```python
from build123d import *

# Parameters (mm, degrees)
SKETCH1_W           = 7.3
SKETCH1_H           = 7.3
BOSS_EXTRUDE1_DEPTH = 1
BOSS_EXTRUDE2_DEPTH = 3
BOSS_EXTRUDE3_DEPTH = 1


with BuildPart() as part:
    # Sketch1 → Boss-Extrude1 (new body)
    with BuildSketch(Plane(origin=(0, 0, 0), x_dir=(1, 0, 0), z_dir=(0, 1, 0))):
        with BuildLine():
            Line((-6, -9), (6, -9))
            ThreePointArc((6, -9), (8.121320344, -8.121320344), (9, -6))
            Line((9, -6), (9, 6))
            ThreePointArc((9, 6), (8.121320344, 8.121320344), (6, 9))
            Line((6, 9), (-6, 9))
            ThreePointArc((-6, 9), (-8.121320344, 8.121320344), (-9, 6))
            Line((-9, 6), (-9, -6))
            ThreePointArc((-9, -6), (-8.121320344, -8.121320344), (-6, -9))
        make_face()
        Rectangle(SKETCH1_W, SKETCH1_H, mode=Mode.SUBTRACT)
    extrude(amount=BOSS_EXTRUDE1_DEPTH)

    # Sketch2 → Boss-Extrude2 (add)
    with BuildSketch(Plane(origin=(0, 1, 0), x_dir=(1, 0, 0), z_dir=(0, 1, 0))):
        with BuildLine():
            Line((-6, -9), (6, -9))
            ThreePointArc((6, -9), (8.121320344, -8.121320344), (9, -6))
            Line((9, -6), (9, 6))
            ThreePointArc((9, 6), (8.121320344, 8.121320344), (6, 9))
            Line((6, 9), (-6, 9))
            ThreePointArc((-6, 9), (-8.121320344, 8.121320344), (-9, 6))
            Line((-9, 6), (-9, -6))
            ThreePointArc((-9, -6), (-8.121320344, -8.121320344), (-6, -9))
        make_face()
        Polygon((-3.05, -3.65), (-3.05, -7.8), (3.05, -7.8), (3.05, -3.65), (3.65, -3.65), (3.65, -3.05), (7.8, -3.05), (7.8, 3.05), (3.65, 3.05), (3.65, 3.65), (3.05, 3.65), (3.05, 7.8), (-3.05, 7.8), (-3.05, 3.65), (-3.65, 3.65), (-3.65, 3.05), (-7.8, 3.05), (-7.8, -3.05), (-3.65, -3.05), (-3.65, -3.65), align=None, mode=Mode.SUBTRACT)
    extrude(amount=BOSS_EXTRUDE2_DEPTH)

    # Sketch3 → Boss-Extrude3 (add)
    with BuildSketch(Plane(origin=(0, 4, 0), x_dir=(1, 0, 0), z_dir=(0, 1, 0))):
        with BuildLine():
            Line((-3.65, -3.05), (-3.65, -3.65))
            Line((-3.65, -3.65), (-3.05, -3.65))
            Line((-3.05, -3.65), (-3.05, -9))
            Line((-3.05, -9), (-6, -9))
            ThreePointArc((-6, -9), (-8.121320344, -8.121320344), (-9, -6))
            Line((-9, -6), (-9, -3.05))
            Line((-9, -3.05), (-3.65, -3.05))
        make_face()
        with BuildLine():
            Line((6, -9), (3.05, -9))
            Line((3.05, -9), (3.05, -3.65))
            Line((3.05, -3.65), (3.65, -3.65))
            Line((3.65, -3.65), (3.65, -3.05))
            Line((3.65, -3.05), (9, -3.05))
            Line((9, -3.05), (9, -6))
            ThreePointArc((9, -6), (8.121320344, -8.121320344), (6, -9))
        make_face()
        with BuildLine():
            Line((3.65, 3.05), (3.65, 3.65))
            Line((3.65, 3.65), (3.05, 3.65))
            Line((3.05, 3.65), (3.05, 9))
            Line((3.05, 9), (6, 9))
            ThreePointArc((6, 9), (8.121320344, 8.121320344), (9, 6))
            Line((9, 6), (9, 3.05))
            Line((9, 3.05), (3.65, 3.05))
        make_face()
        with BuildLine():
            Line((-6, 9), (-3.05, 9))
            Line((-3.05, 9), (-3.05, 3.65))
            Line((-3.05, 3.65), (-3.65, 3.65))
            Line((-3.65, 3.65), (-3.65, 3.05))
            Line((-3.65, 3.05), (-9, 3.05))
            Line((-9, 3.05), (-9, 6))
            ThreePointArc((-9, 6), (-8.121320344, 8.121320344), (-6, 9))
        make_face()
    extrude(amount=BOSS_EXTRUDE3_DEPTH)


solid = part.part
```
The listing builds one solid part. Answer for the finished solid, in the listing's coordinates (mm). A direction names the side the tool comes from. Coordinates: 2 decimals unless noted, no trailing zeros. Loops run counter-clockwise (first coordinate to the right, second up) from the corner with the lowest first, then second, coordinate; pieces in that order, holes last. Notation, with made-up numbers: (3.25, 74.5) -> (33.25, 74.5) arc R18 ccw to (33.25, 80.5) -> close; hole circle Ø8 at (46.5, -21.5). An arc over 180 degrees is marked (long way). Use one line per item in the form item = value. Start each with the question number.
Item 1: The part is cut by section A-A on z = 0.5. Determine the outline of the cut face in (x, y), then the cut area to 3 significant figures.
Item 2: The part is cut by section D-D on y = 0.5. Determine the outline of the cut face in (x, z), then the cut area to 3 significant figures.
Item 3: The mould has two halves that part along X. Classify faces 5 (the face through (0, 2, 9)), 6 (the face through (0, 1, -6)), 7 (the face through (0, 4, 8)), 8 (the face through (-8.1, 2.46, -8.14)): released by +X, released by -X, zero draft, split by the parting line, or undercut.
Item 4: The part is cut by section B-B on y = 4.25. Determine the outline of the cut face in (x, z).
Item 5: Consider L1, parallel to Z at x = 3.25, y = 3.3; L2, parallel to Z at x = 0, y = 1.5; L3, parallel to X at y = 3.25, z = 4.25. Determine where each line is inside the solid, lowest interval first. Write a range as [from, to].
Item 6: The part is cut by section C-C on x = -2. Determine the outline of the cut face in (y, z), then the cut area to 3 significant figures.
Item 7: A tool of negligible diameter and unlimited length cuts with its end or side. For faces 1 (the face through (-0.1, 0.8, 3.65)), 2 (the face through (8, 4, 0)), 3 (the face through (6, 5, -6)), 4 (the face through (6, 3, 3.05)), from which of +Z, -Z, +X, -X, +Y, -Y can it reach the whole face along a straight path? Write none if from no direction.
Item 8: Flat-ended cylindrical pins translate along their axes: pin 1 Ø1.3 at (x, z) = (-0.5, -8) entering from +Y; pin 2 Ø2 at (y, z) = (2.5, 6.5) entering from +X; pin 3 Ø2 at (x, z) = (5.5, 0.5) entering from +Y; pin 4 Ø1.2 at (y, z) = (2, -7.5) entering from -X. Find the tip coordinate at first contact, or state that the pin passes through.
Answer key:
q1.outline = (-9, 0) -> (-3.65, 0) -> (-3.65, 1) -> (-7.8, 1) -> (-7.8, 4) -> (-9, 4) -> close; (3.65, 0) -> (9, 0) -> (9, 4) -> (7.8, 4) -> (7.8, 1) -> (3.65, 1) -> close
q1.area = 17.9 mm2
q2.outline = (-9, -6) arc R3 ccw to (-6, -9) -> (6, -9) arc R3 ccw to (9, -6) -> (9, 6) arc R3 ccw to (6, 9) -> (-6, 9) arc R3 ccw to (-9, 6) -> close; hole (-3.65, -3.65) -> (3.65, -3.65) -> (3.65, 3.65) -> (-3.65, 3.65) -> close
q2.area = 263 mm2
q3.face_5 = zero draft
q3.face_6 = undercut
q3.face_7 = undercut
q3.face_8 = released by -X
q4.outline = (-9, -6) arc R3 ccw to (-6, -9) -> (-3.05, -9) -> (-3.05, -3.65) -> (-3.65, -3.65) -> (-3.65, -3.05) -> (-9, -3.05) -> close; (-9, 3.05) -> (-3.65, 3.05) -> (-3.65, 3.65) -> (-3.05, 3.65) -> (-3.05, 9) -> (-6, 9) arc R3 ccw to (-9, 6) -> close; (3.05, -9) -> (6, -9) arc R3 ccw to (9, -6) -> (9, -3.05) -> (3.65, -3.05) -> (3.65, -3.65) -> (3.05, -3.65) -> close; (3.05, 3.65) -> (3.65, 3.65) -> (3.65, 3.05) -> (9, 3.05) -> (9, 6) arc R3 ccw to (6, 9) -> (3.05, 9) -> close
q5.L1 = [-9, -3.65], [3.65, 9]
q5.L2 = [-9, -7.8], [7.8, 9]
q5.L3 = [-9, -3.05], [3.05, 9]
q6.outline = (0, -9) -> (4, -9) -> (4, -7.8) -> (1, -7.8) -> (1, -3.65) -> (0, -3.65) -> close; (0, 3.65) -> (1, 3.65) -> (1, 7.8) -> (4, 7.8) -> (4, 9) -> (0, 9) -> close
q6.area = 17.9 mm2
q7.face_1 = +Y, -Y
q7.face_2 = +X, -X, +Y
q7.face_3 = +Z, -Z, +X, -X, +Y
q7.face_4 = +Y
q8.pin_1 = 4
q8.pin_2 = 9
q8.pin_3 = 1
q8.pin_4 = -8.86
